Can you work these out from the model? Positions are in its coordinate system, mm. Face numbers are marked on the shaded views. A direction names the side the tool comes from. Round coordinates to 2 decimals unless told otherwise and drop trailing zeros. Write each loop counter-clockwise with the first axis right and the second up, starting at its lowest first coordinate (ties: lowest second). Pieces come first, ordered by that corner, then holes. Notation, with made-up numbers: (70.5, 12.25) -> (121.5, 12.25) arc R18 cw to (121.5, 22.25) -> close; hole circle Ø10 at (5.25, 36). An arc over 180 degrees is marked (long way). Use CSV: the item, a comma, the result in double quotes.
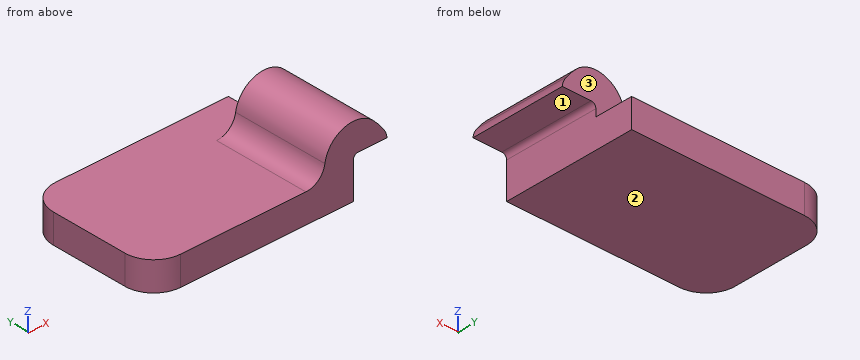
```python
from build123d import *

# Parameters (mm, degrees)
F1_DEPTH = 19.05
F4_DEPTH = 63.5


with BuildPart() as f1:
    # F0 (on Top) → F1 (new body)
    with BuildSketch(Plane.XY):
        with BuildLine():
            Line((-139.7, -63.5), (-25.4, -63.5))
            Line((-25.4, -63.5), (-25.4, 25.4))
            Line((-25.4, 25.4), (-139.7, 25.4))
            ThreePointArc((-139.7, 25.4), (-153.170384, 19.820384), (-158.75, 6.35))
            Line((-158.75, 6.35), (-158.75, -44.45))
            ThreePointArc((-158.75, -44.45), (-153.170384, -57.920384), (-139.7, -63.5))
        make_face()
    extrude(amount=F1_DEPTH)

    # F3 (on offset) → F4 (join)
    with BuildSketch(Plane.XZ.offset(63.5)):
        with BuildLine():
            Line((-56.79078, 19.05), (-25.4, 19.05))
            Line((-25.4, 19.05), (-25.4, 23.8125))
            ThreePointArc((-25.4, 23.8125), (-24.470064, 26.057564), (-22.225, 26.9875))
            Line((-22.225, 26.9875), (-3.175, 26.9875))
            ThreePointArc((-3.175, 26.9875), (-4.166839, 30.646295), (-6.194382, 33.849356))
            ThreePointArc((-6.194382, 33.849356), (-8.443828, 36.717161), (-10.932128, 39.380368))
            ThreePointArc((-10.932128, 39.380368), (-30.643815, 45.301563), (-44.234468, 29.845))
            ThreePointArc((-44.234468, 29.845), (-48.511393, 22.119748), (-56.79078, 19.05))
        make_face()
    extrude(amount=-F4_DEPTH)


solid = f1.part
```
Q1. Suppose I cut it at C-C (x = -125). Write out the boundary of the cut face in (y, z), and give its area (3 significant figures).
Resolved:
outline,"(-63.5, 0) -> (25.4, 0) -> (25.4, 19.05) -> (-63.5, 19.05) -> close"
area,"1,690 mm^2"
Q2. Please list where these lines run through material, in increasing order: probe 1 along Z at (x, y) = (-76.5, -14); probe 2 along X at (y, z) = (-21.5, 11.5).
Resolved:
probe 1,"z = 0 to 19.05"
probe 2,"x = -158.75 to -25.4"
Q3. On a 3-axis mill with a long thin cutter (end or side, diameter ignored), from which of +Z, -Z, +X, -X, +Y, -Y can I reach the whole of each face in a straight line? I mean the marked faces 1, 2 and 3. Say none if no direction works.
Resolved:
face 1,"-Z, +X, +Y, -Y"
face 2,"-Z, +X, -X, +Y, -Y"
face 3,"+Z, +X, -X, +Y"
Q4. Will these pins go through, and if not, where does the flat tip stop? P1, Ø8, axis at x = -93.5, y = -40.5, coming from the +Z side; P2, Ø12, axis at y = 8.5, z = 25.5, coming from the +X side; P3, Ø9.5, axis at x = -17, y = -29.5, coming from the -Z side; P4, Ø19, axis at y = -21.5, z = 11.5, coming from the +X side.
Resolved:
P1,"stops at z = 19.05"
P2,"passes through"
P3,"stops at z = 26.99"
P4,"stops at x = -25.4"
Q5. Suppose I cut it at B-B (z = 7). Write out the boundary of the cut face in (x, y).
Resolved:
outline,"(-158.75, -44.45) arc R19.05 ccw to (-139.7, -63.5) -> (-25.4, -63.5) -> (-25.4, 25.4) -> (-139.7, 25.4) arc R19.05 ccw to (-158.75, 6.35) -> close"
